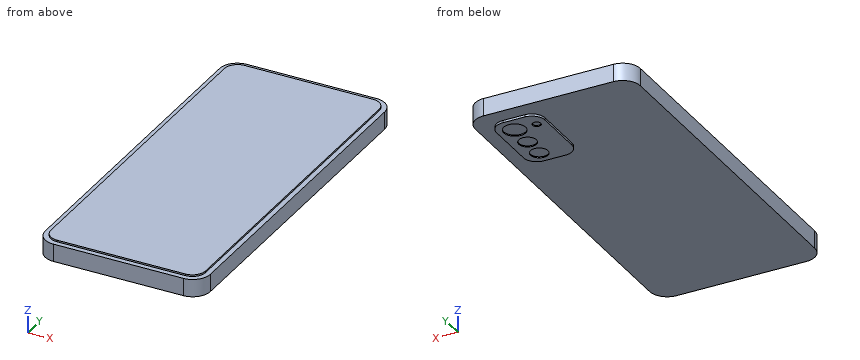
```python
from build123d import *

# Parameters (mm, degrees)
SKETCH1_W           = 75
SKETCH1_H           = 165
BOSS_EXTRUDE1_DEPTH = 8
FILLET1_R           = 8
SKETCH2_W           = 22
SKETCH2_H           = 35
BOSS_EXTRUDE2_DEPTH = 1
FILLET2_R           = 6
SKETCH3_R           = 5
SKETCH3_R_2         = 4
SKETCH3_R_3         = 1.859320818
CUT_EXTRUDE1_DEPTH  = 0.5
SKETCH4_W           = 70.313708498
SKETCH4_H           = 160.313708498
BOSS_EXTRUDE3_DEPTH = 0.75
FILLET3_R           = 6


with BuildPart() as part:
    # Sketch1 → Boss-Extrude1 (new body)
    with BuildSketch(Plane.XY):
        Rectangle(SKETCH1_W, SKETCH1_H)
    extrude(amount=BOSS_EXTRUDE1_DEPTH)

    # Fillet1
    fillet1_edges = [part.edges().sort_by_distance(p)[0] for p in [
        (37.5, -82.5, 4),
        (-37.5, -82.5, 4),
        (-37.5, 82.5, 4),
        (37.5, 82.5, 4),
    ]]
    fillet(fillet1_edges, radius=FILLET1_R)

    # Sketch2 → Boss-Extrude2 (add)
    with BuildSketch(Plane(origin=(0, 0, 0), x_dir=(-1, 0, 0), z_dir=(0, 0, -1))):
        with Locations((-19.5, 58)):
            Rectangle(SKETCH2_W, SKETCH2_H)
    extrude(amount=BOSS_EXTRUDE2_DEPTH)

    # Fillet2
    fillet2_edges = [part.edges().sort_by_distance(p)[0] for p in [
        (8.5, 40.5, -0.5),
        (8.5, 75.5, -0.5),
        (30.5, 75.5, -0.5),
        (30.5, 40.5, -0.5),
    ]]
    fillet(fillet2_edges, radius=FILLET2_R)

    # Sketch3 → Cut-Extrude1 (cut)
    with BuildSketch(Plane(origin=(0, 0, -1), x_dir=(-1, 0, 0), z_dir=(0, 0, -1))):
        with Locations((-23.043680303, 68)):
            Circle(SKETCH3_R)
        with Locations((-23.043680303, 57)):
            Circle(SKETCH3_R_2)
        with Locations((-23.043680303, 47)):
            Circle(SKETCH3_R_2)
        with Locations((-13.043680303, 68)):
            Circle(SKETCH3_R_3)
    extrude(amount=-CUT_EXTRUDE1_DEPTH, mode=Mode.SUBTRACT)

    # Sketch4 → Boss-Extrude3 (add)
    with BuildSketch(Plane.XY.offset(8)):
        Rectangle(SKETCH4_W, SKETCH4_H)
    extrude(amount=BOSS_EXTRUDE3_DEPTH)

    # Fillet3
    fillet3_edges = [part.edges().sort_by_distance(p)[0] for p in [
        (-35.156854249, 80.156854249, 8.375),
        (-35.156854249, -80.156854249, 8.375),
        (35.156854249, -80.156854249, 8.375),
        (35.156854249, 80.156854249, 8.375),
    ]]
    fillet(fillet3_edges, radius=FILLET3_R)


solid = part.part
```
Geometry: final body of the model. Coordinates: model frame, mm. Give positions to 0.01 mm unless a question says otherwise; leave off trailing zeros. Loops run counter-clockwise (first coordinate to the right, second up) from the corner with the lowest first, then second, coordinate; pieces in that order, holes last. Notation, with made-up numbers: (-16, 86.5) - (28, 86.5) arc R19 cw to (28, 103.5) - close; hole circle Ø3 at (70.5, 19.25). An arc over 180 degrees is marked (long way). Answer as CSV lines item,"result". Start each with the question number.
(1) Ray query, line 1 along Z through (x, y) = (-13, -54.5); line 2 along X through (y, z) = (-38.5, 8.25); line 3 along Y through (x, z) = (33.5, 3.75). Return the intervals inside material, ascending. Write a range as [from, to].
(2) Pin query (flat end, axial travel): P1, Ø0.5, axis at x = 17.5, z = -0.5, coming from the +Y side; P2, Ø3, axis at x = 22, y = -20.5, coming from the -Z side; P3, Ø1.1, axis at x = 14, y = 68.5, coming from the -Z side. Return the tip coordinate at first contact, or that it passes through.
(3) Section query C-C (y = 68). Output: boundary loops of the cut face in (x, z).
(4) Section query A-A (y = 6). Output: boundary loops of the cut face in (x, z).
(5) Section query B-B (x = -12.5). Output: boundary loops of the cut face in (y, z), and give its area (3 significant figures).
Worked answers:
1,line 1,"z = [0, 8.75]"
1,line 2,"x = [-35.16, 35.16]"
1,line 3,"y = [-81.43, 81.43]"
2,P1,"stops at y = 75.5"
2,P2,"stops at z = 0"
2,P3,"stops at z = -0.5"
3,outline,"(-37.5, 0) - (8.5, 0) - (8.5, -1) - (11.18, -1) - (11.18, -0.5) - (14.9, -0.5) - (14.9, -1) - (18.04, -1) - (18.04, -0.5) - (28.04, -0.5) - (28.04, -1) - (30.5, -1) - (30.5, 0) - (37.5, 0) - (37.5, 8) - (35.16, 8) - (35.16, 8.75) - (-35.16, 8.75) - (-35.16, 8) - (-37.5, 8) - close"
4,outline,"(-37.5, 0) - (37.5, 0) - (37.5, 8) - (35.16, 8) - (35.16, 8.75) - (-35.16, 8.75) - (-35.16, 8) - (-37.5, 8) - close"
5,outline,"(-82.5, 0) - (82.5, 0) - (82.5, 8) - (80.16, 8) - (80.16, 8.75) - (-80.16, 8.75) - (-80.16, 8) - (-82.5, 8) - close"
5,area,"1,440 mm^2"
